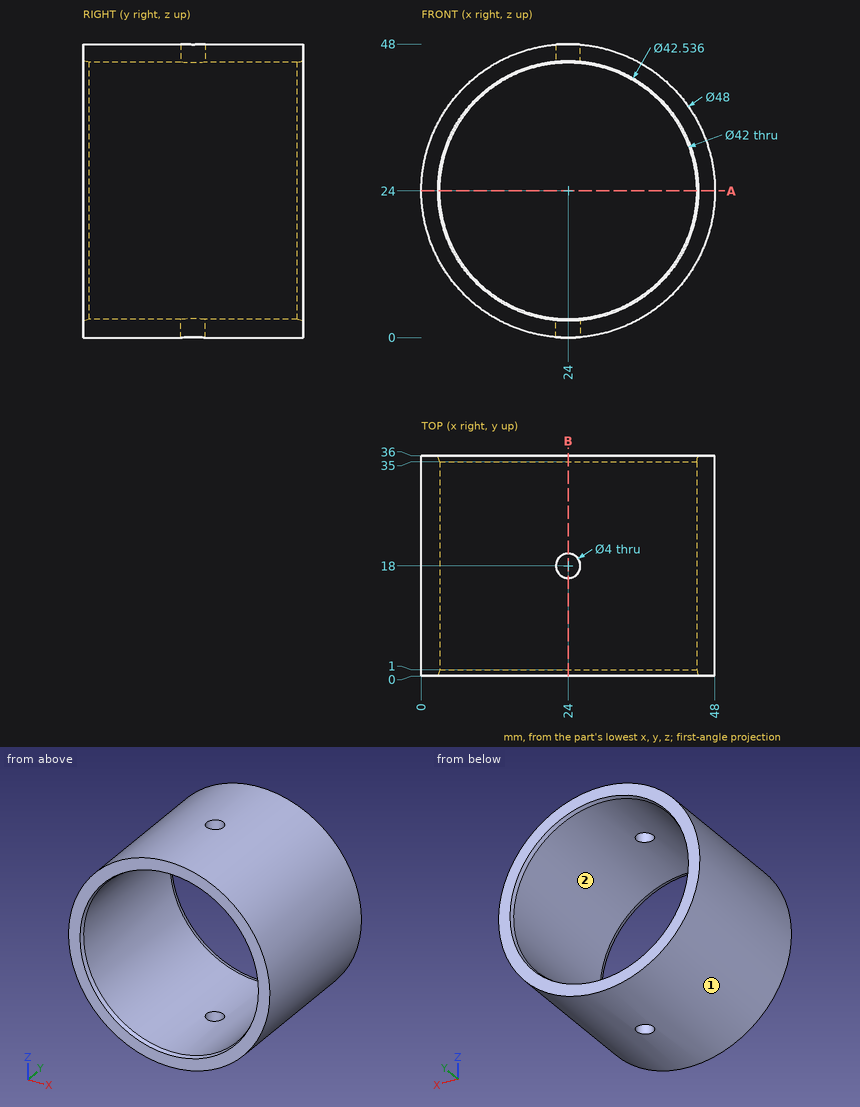
Print and shaded views of the part. All mm, measured from the part's lowest x, y and z. Coordinates: 2 decimals unless noted, no trailing zeros. Order: outer loops, then holes, each group sorted by start corner. A loop starts at its lowest first (then second) coordinate and runs counter-clockwise, first axis right, second up. Notation, with made-up numbers: M -15,75 L -3,75 A12 ccw -3,97 Z; hole C 29,23 d1. An arc over 180 degrees is marked long. One line per question, with ' | ' between items. Start each with the question number.
Q1. Flat gauge pins, fed straight in: pin 1 Ø2 at (x, y) = (32.5, 28.5) entering from -Z; pin 2 Ø2 at (y, z) = (8.5, 42) entering from +X; pin 3 Ø10 at (y, z) = (30, 26) entering from +X; pin 4 Ø4.5 at (x, y) = (24, 18) entering from -Z. Where does each tip first touch, or does it go through?
Q2. Probe L1, parallel to X at y = 15, z = 24; L2, parallel to X at y = 3, z = 42.5; L3, parallel to Z at x = 20, y = 32. List the from-to ranges inside material, lowest first. Write a range as from..to.
Q3. Two-plate mould, pull along Z, no slides. Class the marked faces 1 and 2: +Z half, -Z half, draft (parallel to the pull), parting line (faces both ways), or undercut.
Q4. Saw through at B-B (x = 24). List the corners of the cut face in (y, z).
Q5. Saw through at A-A (z = 24). List the corners of the cut face in (x, y), then the cut area to 3 significant figures.
Check values:
1) pin 1: stops at z = 1.2 | pin 2: stops at x = 40.94 | pin 3: stops at x = 48 | pin 4: stops at z = 0
2) L1: x = 0..3, 45..48 | L2: x = 8.71..14.06, 33.94..39.29 | L3: z = 0.34..3.38, 44.62..47.66
3) face 1: parting line | face 2: undercut
4) outline: M 0,0 L 16,0 L 16,3 L 1,3 L 0,2.73 Z; M 0,45.27 L 1,45 L 16,45 L 16,48 L 0,48 Z; M 20,0 L 36,0 L 36,2.73 L 35,3 L 20,3 Z; M 20,45 L 35,45 L 36,45.27 L 36,48 L 20,48 Z
5) outline: M 0,0 L 2.73,0 L 3,1 L 3,35 L 2.73,36 L 0,36 Z; M 45,1 L 45.27,0 L 48,0 L 48,36 L 45.27,36 L 45,35 Z | area: 215 mm2
